CAD build for the part. Positions are in the model's coordinates, mm. A direction names the side the tool comes from. Round coordinates to 2 decimals unless told otherwise and drop trailing zeros. Order: outer loops, then holes, each group sorted by start corner. A loop starts at its lowest first (then second) coordinate and runs counter-clockwise, first axis right, second up.
```python
from build123d import *

# Parameters (mm, degrees)
BOSS_EXTRUDE1_DEPTH = 12.7
SKETCH2_W           = 10.16
SKETCH2_H           = 38.1
SKETCH2_W_2         = 6.35
SKETCH2_H_2         = 12.7
BOSS_EXTRUDE2_DEPTH = 10.16
BOSS_EXTRUDE3_DEPTH = 12.7
CUT_EXTRUDE1_DEPTH  = 15.24
FILLET2_R           = 2.54
FILLET4_R           = 1.27
BOSS_EXTRUDE4_DEPTH = 3.81


with BuildPart() as part:
    # Sketch1 → Boss-Extrude1 (new body)
    with BuildSketch(Plane(origin=(0, 0, 0), x_dir=(1, 0, 0), z_dir=(0, 1, 0))):
        Polygon((-38.1, 76.2), (38.1, 76.2), (76.2, 38.1), (76.2, -38.1), (38.1, -76.2), (-38.1, -76.2), (-76.2, -38.1), (-76.2, 38.1), align=None)
    extrude(amount=BOSS_EXTRUDE1_DEPTH)

    # Sketch2 → Boss-Extrude2 (add)
    with BuildSketch(Plane(origin=(0, 12.7, 0), x_dir=(1, 0, 0), z_dir=(0, 1, 0))):
        Rectangle(SKETCH2_W, SKETCH2_H)
        with Locations((61.595, 0)):
            Rectangle(SKETCH2_W_2, SKETCH2_H)
        with Locations((-65.405, 12.7)):
            Rectangle(SKETCH2_W_2, SKETCH2_H_2)
        with Locations((-65.405, -12.7)):
            Rectangle(SKETCH2_W_2, SKETCH2_H_2)
    extrude(amount=BOSS_EXTRUDE2_DEPTH)

    # Sketch4 → Boss-Extrude3 (add)
    with BuildSketch(Plane(origin=(0, 12.7, 0), x_dir=(1, 0, 0), z_dir=(0, 1, 0))):
        Polygon((-69.85, -44.45), (69.85, -44.45), (38.1, -76.2), (-38.1, -76.2), align=None)
    extrude(amount=BOSS_EXTRUDE3_DEPTH)

    # Sketch5 → Cut-Extrude1 (cut)
    with BuildSketch(Plane(origin=(0, 25.4, 0), x_dir=(1, 0, 0), z_dir=(0, 1, 0))):
        Polygon((11.557, -58.721300535), (18.829335275, -58.721300535), (18.829335275, -44.45), (22.639335275, -44.45), (22.639335275, -62.531300535), (11.557, -62.531300535), (11.557, -66.37376468), (-11.557, -66.37376468), (-11.557, -53.67376468), (11.557, -53.67376468), align=None)
    extrude(amount=-CUT_EXTRUDE1_DEPTH, mode=Mode.SUBTRACT)

    # Fillet2
    fillet2_edges = [part.edges().sort_by_distance(p)[0] for p in [
        (-53.975, 25.4, 60.325),
        (0, 25.4, 76.2),
        (53.975, 25.4, 60.325),
        (46.244667637, 25.4, 44.45),
        (-25.510332363, 25.4, 44.45),
        (17.098167637, 25.4, 62.531300535),
        (22.639335275, 25.4, 53.490650267),
        (18.829335275, 25.4, 51.585650267),
        (15.193167637, 25.4, 58.721300535),
    ]]
    fillet(fillet2_edges, radius=FILLET2_R)

    # Fillet4
    fillet4_edges = [part.edges().sort_by_distance(p)[0] for p in [
        (5.08, 22.86, 0),
        (0, 22.86, -19.05),
        (-5.08, 22.86, 0),
        (0, 22.86, 19.05),
        (58.42, 22.86, 0),
        (61.595, 22.86, 19.05),
        (64.77, 22.86, 0),
        (61.595, 22.86, -19.05),
        (-62.23, 22.86, -12.7),
        (-65.405, 22.86, -19.05),
        (-68.58, 22.86, -12.7),
        (-65.405, 22.86, -6.35),
        (-62.23, 22.86, 12.7),
        (-65.405, 22.86, 6.35),
        (-68.58, 22.86, 12.7),
        (-65.405, 22.86, 19.05),
    ]]
    fillet(fillet4_edges, radius=FILLET4_R)

    # Sketch8 → Boss-Extrude4 (add)
    with BuildSketch(Plane(origin=(18.829335275, 0, 0), x_dir=(0, 0, -1), z_dir=(1, 0, 0))):
        Polygon((-58.721300535, 10.16), (-44.45, 12.7), (-44.45, 10.16), align=None)
    extrude(amount=BOSS_EXTRUDE4_DEPTH)


solid = part.part
```
1. Tool access for faces 5 (the face through (-68.58, 17, 13)), 6 (the face through (-26, 18, 44.45)), 7 (the face through (64.77, 17, 0)), 8 (the face through (-65, 17, -6.35)), 9 (the face through (11.557, 18, 56)): list every direction of +Z, -Z, +X, -X, +Y, -Y with a clear straight run to the whole face (end or side of a thin tool).
2. Cut at C-C, the plane y = 7. Write the cut outline in (x, z).
3. Cut at B-B, the plane z = -0.5. Write the cut outline in (x, y).
4. Mould opens along X. For faces 1 (the face through (0, 17, -19.05)), 2 (the face through (11.557, 18, 64)), 3 (the face through (5.08, 17, 0)), 4 (the face through (56.9, 6.3, -57.4)) say: released by +X, released by -X, zero draft, split by the parting line, or undercut.
5. Drill centre lines: line 1 (X direction, y = 23.25, z = 54); line 2 (Y direction, x = -27, z = -35.5); line 3 (X direction, y = 18.75, z = -2.5). Where is each one in solid material? Low to high.
6. Cut at D-D, the plane z = -62.5. Write the cut outline in (x, y), and give its area (3 significant figures).
7. Cut at A-A, the plane x = 27. Write the cut outline in (y, z).
8. Pin check, flat tips, straight feed: P1, Ø2, axis at x = -12.5, z = 20.5, coming from the +Y side; P2, Ø7, axis at y = 16.5, z = -13, coming from the -X side; P3, Ø2.5, axis at y = 15, z = -1, coming from the +X side. Stop position of each tip, or through.
Outcome:
1. face 5: -Z, -X, +Y
1. face 6: +X, -X, +Y
1. face 7: -Z, +X, +Y
1. face 8: -X, +Y
1. face 9: +Y
2. outline: (-76.2, -38.1) - (-38.1, -76.2) - (38.1, -76.2) - (76.2, -38.1) - (76.2, 38.1) - (38.1, 76.2) - (-38.1, 76.2) - (-76.2, 38.1) - close
3. outline: (-76.2, 0) - (76.2, 0) - (76.2, 12.7) - (64.77, 12.7) - (64.77, 21.59) arc R1.27 ccw to (63.5, 22.86) - (59.69, 22.86) arc R1.27 ccw to (58.42, 21.59) - (58.42, 12.7) - (5.08, 12.7) - (5.08, 21.59) arc R1.27 ccw to (3.81, 22.86) - (-3.81, 22.86) arc R1.27 ccw to (-5.08, 21.59) - (-5.08, 12.7) - (-76.2, 12.7) - close
4. face 1: zero draft
4. face 2: undercut
4. face 3: undercut
4. face 4: released by +X
5. line 1: x = -60.26 to -11.56, 11.56 to 18.8, 22.67 to 60.26
5. line 2: y = 0 to 12.7
5. line 3: x = -5.08 to 5.08, 58.42 to 64.77
6. outline: (-51.8, 0) - (51.8, 0) - (51.8, 12.7) - (-51.8, 12.7) - close
6. area: 1,320 mm2
7. outline: (0, -76.2) - (12.7, -76.2) - (12.7, 44.45) - (22.86, 44.45) arc R2.54 ccw to (25.4, 46.99) - (25.4, 73.66) arc R2.54 ccw to (22.86, 76.2) - (0, 76.2) - close
8. P1: stops at y = 12.7
8. P2: stops at x = -68.58
8. P3: stops at x = 64.77
